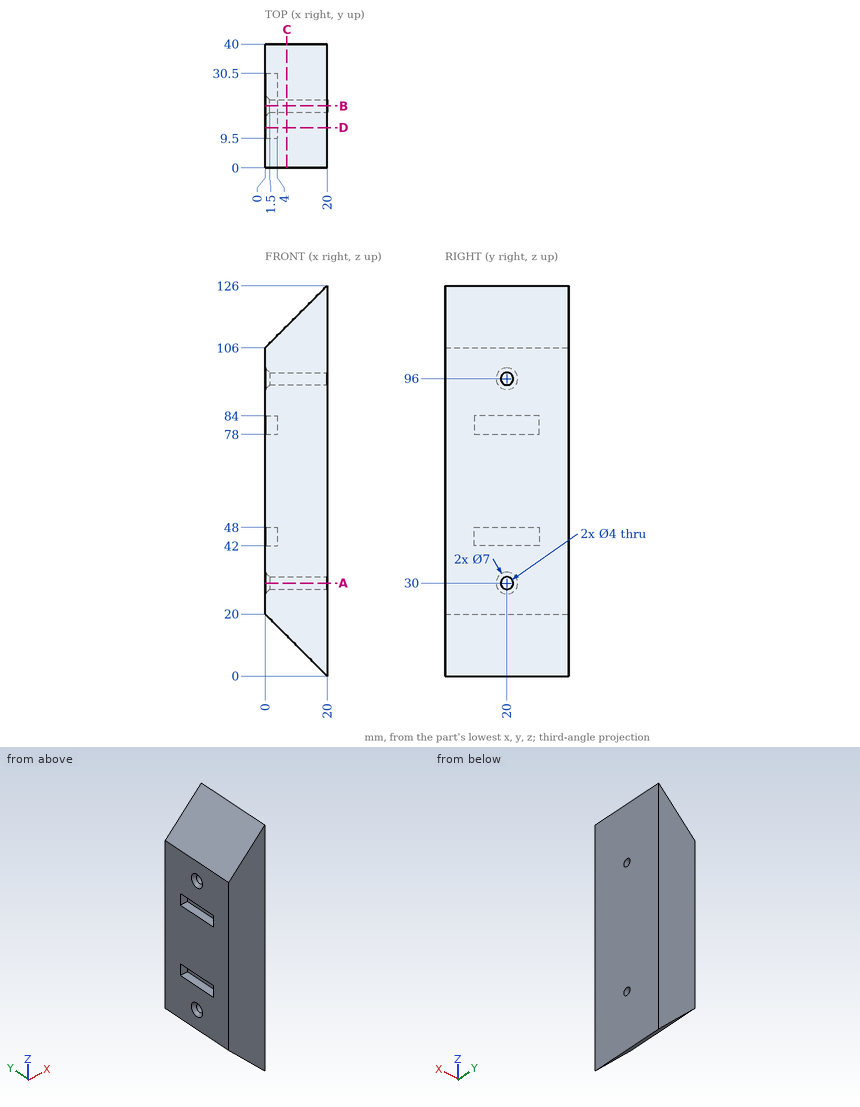
Study the drawing (mm; zero at the part's minimum x, y, z) and answer. Round coordinates to 2 decimals unless told otherwise and drop trailing zeros. Write each loop counter-clockwise with the first axis right and the second up, starting at its lowest first coordinate (ties: lowest second). Pieces come first, ordered by that corner, then holes.
1) A cutting plane is placed at C-C (x = 7). Give the vertices of the cut face in (y, z).
2) A cutting plane is placed at D-D (y = 13). Give the vertices of the cut face in (x, z), plus the area to 3 significant figures.
3) Given pin 1 Ø5 at (y, z) = (29, 111.5) entering from -X; pin 2 Ø4.5 at (x, y) = (2, 16) entering from +Z; pin 3 Ø4.5 at (x, y) = (1, 21) entering from -Z, each flat-ended and moving along its own axis, determine where each tip first touches the part or whether it passes through.
4) A cutting plane is placed at B-B (y = 20). Give the vertices of the cut face in (x, z).
5) A cutting plane is placed at A-A (z = 30). Give the vertices of the cut face in (x, y), plus the area to 3 significant figures.
6) Straight lines are drawn through the part: line 1 (Z direction, x = 8.5, y = 20); line 2 (Z direction, x = 14.25, y = 20); line 3 (Y direction, x = 10, z = 96). For each, find the intervals that lie inside material, in ascending order.
Completed:
1. outline: (0, 13) - (40, 13) - (40, 113) - (0, 113) - close; hole circle Ø4 at (20, 30); hole circle Ø4 at (20, 96)
2. outline: (0, 20) - (20, 0) - (20, 126) - (0, 106) - (0, 84) - (4, 84) - (4, 78) - (0, 78) - (0, 48) - (4, 48) - (4, 42) - (0, 42) - close
2. area: 2,070 mm2
3. pin 1: stops at x = 3
3. pin 2: stops at z = 110.25
3. pin 3: stops at z = 16.75
4. outline: (0, 20) - (20, 0) - (20, 28) - (1.5, 28) - (0, 26.5) - close; (0, 33.5) - (1.5, 32) - (20, 32) - (20, 94) - (1.5, 94) - (0, 92.5) - (0, 84) - (4, 84) - (4, 78) - (0, 78) - (0, 48) - (4, 48) - (4, 42) - (0, 42) - close; (0, 99.5) - (1.5, 98) - (20, 98) - (20, 126) - (0, 106) - close
5. outline: (0, 0) - (20, 0) - (20, 18) - (1.5, 18) - (0, 16.5) - close; (0, 23.5) - (1.5, 22) - (20, 22) - (20, 40) - (0, 40) - close
5. area: 718 mm2
6. line 1: z = 11.5 to 28, 32 to 94, 98 to 114.5
6. line 2: z = 5.75 to 28, 32 to 94, 98 to 120.25
6. line 3: y = 0 to 18, 22 to 40
